The model under review builds one solid part; all positions refer to its coordinate system, in mm. A direction names the side the tool comes from. Round coordinates to 2 decimals unless told otherwise and drop trailing zeros. Order: outer loops, then holes, each group sorted by start corner. A loop starts at its lowest first (then second) coordinate and runs counter-clockwise, first axis right, second up. Notation, with made-up numbers: M -31,-17 L 11,-17 A12 ccw 11,5 Z; hole C -35,71.25 d11. An arc over 180 degrees is marked long. Answer as a JSON object with one key per item and string values. Group by question number.
1. Machinability: for faces 1 (the face through (38, 0, -80)), 2 (the face through (-29.97, 1.32, -9.86)), 3 (the face through (1, 10, -64)), 4 (the face through (-45, 0, -100)), which of the approach directions +Z, -Z, +X, -X, +Y, -Y give a long, thin tool a straight path to every point of the face, cutting with its end or side? Answer none if there is none.
2. Add section D-D on z = -51. State the section outline as (x, y) points, and give its area (3 significant figures).
3. Add section A-A on x = 28. State the section outline as (y, z) points.
4. Add section C-C on x = 0. State the section outline as (y, z) points.
5. To check wall thickness, follow probe 1 along Y at (x, z) = (23, -44); probe 2 along X at (y, z) = (4, -34); probe 3 along Z at (x, y) = (-16, 2). State the ranges of each line that lie inside material, in increasing order. Write a range as [from, to].
6. Add section B-B on y = 0. State the section outline as (x, z) points, and give its area (3 significant figures).
7. Mouldability with a two-part tool opening along X and no side actions: class faces 5 (the face through (1, 0, -90)), 6 (the face through (0, -13, -20)), 7 (the face through (25, 0, -50)), 8 (the face through (45, 0, -100)) as released by +X, released by -X, zero draft, split by the parting line, or undercut.
8. Clearance check with flat-ended pins moving along their axes: P1, Ø1, axis at x = 0.5, z = -78.5, coming from the -Y side; P2, Ø6, axis at x = -42.5, y = -5, coming from the +Z side; P3, Ø12, axis at y = -3.5, z = -22, coming from the +X side. State where each tip first meets the part, or that it passes through.
```python
from build123d import *

# Parameters (mm, degrees)
SKETCH1_R           = 30
BOSS_EXTRUDE1_DEPTH = 20
SKETCH3_W           = 50
SKETCH3_H           = 20
BOSS_EXTRUDE2_DEPTH = 60
SKETCH4_W           = 100
SKETCH4_H           = 20
BOSS_EXTRUDE3_DEPTH = 10
SKETCH5_W           = 5
SKETCH5_H           = 20
BOSS_EXTRUDE4_DEPTH = 20


with BuildPart() as part:
    # Sketch1 → Boss-Extrude1 (new body)
    with BuildSketch(Plane.XY):
        Circle(SKETCH1_R)
    extrude(amount=-BOSS_EXTRUDE1_DEPTH)

    # Sketch3 → Boss-Extrude2 (add)
    with BuildSketch(Plane(origin=(0, 0, -20), x_dir=(-1, 0, 0), z_dir=(0, 0, -1))):
        Rectangle(SKETCH3_W, SKETCH3_H)
    extrude(amount=BOSS_EXTRUDE2_DEPTH)

    # Sketch4 → Boss-Extrude3 (add)
    with BuildSketch(Plane(origin=(0, 0, -80), x_dir=(-1, 0, 0), z_dir=(0, 0, -1))):
        Rectangle(SKETCH4_W, SKETCH4_H)
    extrude(amount=BOSS_EXTRUDE3_DEPTH)

    # Sketch5 → Boss-Extrude4 (add)
    with BuildSketch(Plane(origin=(0, 0, -90), x_dir=(-1, 0, 0), z_dir=(0, 0, -1))):
        with Locations((-47.5, 0)):
            Rectangle(SKETCH5_W, SKETCH5_H)
        with Locations((47.5, 0)):
            Rectangle(SKETCH5_W, SKETCH5_H)
    extrude(amount=BOSS_EXTRUDE4_DEPTH)


solid = part.part
```
Recorded:
{
 "1": {"face 1": "+X, +Y, -Y", "face 2": "+Z", "face 3": "-Z, +X, -X, +Y", "face 4": "-Z, +Y, -Y"},
 "2": {"outline": "M -25,-10 L 25,-10 L 25,10 L -25,10 Z", "area": "1,000 mm²"},
 "3": {"outline": "M -10.77,-20 L 10.77,-20 L 10.77,0 L -10.77,0 Z; M -10,-90 L 10,-90 L 10,-80 L -10,-80 Z"},
 "4": {"outline": "M -30,-20 L -10,-20 L -10,-90 L 10,-90 L 10,-20 L 30,-20 L 30,0 L -30,0 Z"},
 "5": {"probe 1": "y = [-10, 10]", "probe 2": "x = [-25, 25]", "probe 3": "z = [-90, 0]"},
 "6": {"outline": "M -50,-110 L -45,-110 L -45,-90 L 45,-90 L 45,-110 L 50,-110 L 50,-80 L 25,-80 L 25,-20 L 30,-20 L 30,0 L -30,0 L -30,-20 L -25,-20 L -25,-80 L -50,-80 Z", "area": "5,400 mm²"},
 "7": {"face 5": "undercut", "face 6": "zero draft", "face 7": "released by +X", "face 8": "undercut"},
 "8": {"P1": "stops at y = -10", "P2": "stops at z = -80", "P3": "stops at x = 30"}
}
